Study the drawing (mm; zero at the part's minimum x, y, z) and answer. Coordinates: 2 decimals unless noted, no trailing zeros. Loops run counter-clockwise (first coordinate to the right, second up) from the corner with the lowest first, then second, coordinate; pieces in that order, holes last. Notation, with made-up numbers: (20.25, 86) -> (24.25, 86) arc R9 cw to (24.25, 92) -> close; hole circle Ø9 at (-20.5, 6.25). An arc over 180 degrees is marked (long way). Answer as a JSON object with one key per item and string values. Group by question number.
Q1. Each of these flat-tipped pins is pushed along its axis until it touches: P1, Ø12, axis at x = 62, z = 38, coming from the +Y side; P2, Ø6, axis at y = 10.5, z = 120, coming from the -X side; P3, Ø1.2, axis at x = 108, y = 16, coming from the -Z side; P4, Ø1.3, axis at y = 7.5, z = 113.5, coming from the +X side. Where does it stop, or does it pass through?
Q2. Straight lines are drawn through the part: line 1 along Z through (x, y) = (106.5, 4.5); line 2 along Y through (x, z) = (203, 69); line 3 along X through (y, z) = (6.75, 113). For each, find the intervals that lie inside material, in ascending order. Write a range as [from, to].
Q3. The part is cut by section C-C on y = 19.5. Write down the section's boundary in (x, z), and give its area (3 significant figures).
Q4. The part is cut by section D-D on z = 26. Write down the section's boundary in (x, y).
Q5. The part is cut by section A-A on x = 174.5. Write down the section's boundary in (y, z).
Q6. The part is cut by section B-B on z = 99. Write down the section's boundary in (x, y), and give its area (3 significant figures).
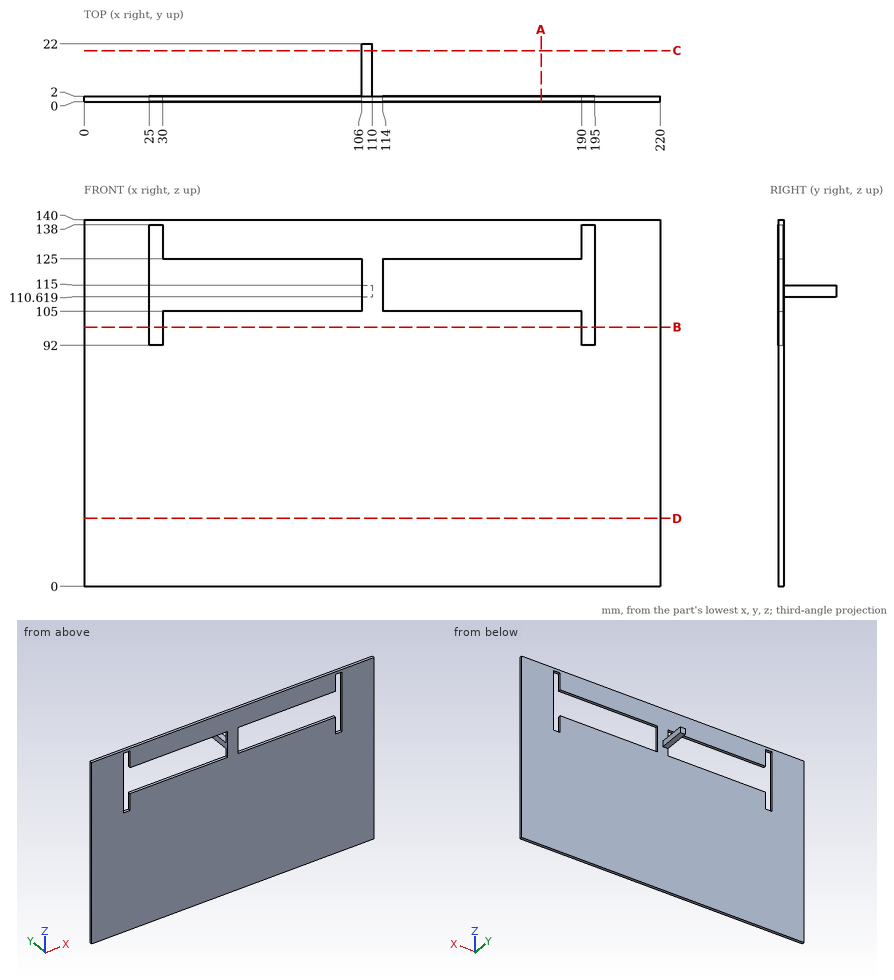
Final values:
{
 "1": {"P1": "stops at y = 2", "P2": "passes through", "P3": "stops at z = 110.62", "P4": "stops at x = 110"},
 "2": {"line 1": "z = [110.62, 115]", "line 2": "y = [0, 2]", "line 3": "x = [106, 110]"},
 "3": {"outline": "(106, 110.62) -> (110, 110.62) -> (110, 115) -> (106, 115) -> close", "area": "17.5 mm2"},
 "4": {"outline": "(0, 0) -> (220, 0) -> (220, 2) -> (0, 2) -> close"},
 "5": {"outline": "(0, 0) -> (2, 0) -> (2, 105) -> (0, 105) -> close; (0, 125) -> (2, 125) -> (2, 140) -> (0, 140) -> close"},
 "6": {"outline": "(0, 0) -> (25, 0) -> (25, 2) -> (0, 2) -> close; (30, 0) -> (190, 0) -> (190, 2) -> (30, 2) -> close; (195, 0) -> (220, 0) -> (220, 2) -> (195, 2) -> close", "area": "420 mm2"}
}
